For this review, take the finished solid that the model builds, in its own axes (mm). A direction names the side the tool comes from. Coordinates: 2 decimals unless noted, no trailing zeros. Order: outer loops, then holes, each group sorted by start corner. A loop starts at its lowest first (then second) coordinate and runs counter-clockwise, first axis right, second up.
from build123d import *

# Parameters (mm, degrees)
CORTAR_EXTRUIR4_DEPTH      = 312.012057644
SALIENTE_EXTRUIR1_START    = -30
CROQUIS4_R                 = 67.5
SALIENTE_EXTRUIR1_DEPTH    = 30
SALIENTE_EXTRUIR2_START    = 2
CROQUIS5_R                 = 58
CROQUIS5_R_2               = 50.227847336
CROQUIS5_R_3               = 2.860878396
SALIENTE_EXTRUIR2_DEPTH    = 2
CROQUIS6_R                 = 58
SALIENTE_EXTRUIR3_DEPTH    = 73
CORTAR_EXTRUIR5_DEPTH      = 315.148452169
CORTAR_EXTRUIR5_DEPTH_BACK = 315.148452169
CROQUIS7_W                 = 212.825411986
CROQUIS7_H                 = 84.990442804


with BuildPart() as part:
    # Croquis2 → Revolución1 (revolve)
    with BuildSketch(Plane.XY):
        Polygon((0, 0), (-67.5, 0), (-67.5, 26.689315597), (-58, 80), (-58, 296), (0, 296), align=None)
    revolve(axis=Axis((0, 296, 0), (0, -1, 0)))

    # Croquis3 → Cortar-Extruir4 (cut, through all)
    with BuildSketch(Plane(origin=(0, 296, 0), x_dir=(1, 0, 0), z_dir=(0, 1, 0))):
        Polygon((0, 58), (-8.909431544, 66.909431544), (8.909431544, 66.909431544), align=None)
        Polygon((66.909431544, -8.909431544), (58, 0), (66.909431544, 8.909431544), align=None)
        Polygon((-8.909431544, -66.909431544), (0, -58), (8.909431544, -66.909431544), align=None)
        Polygon((-66.909431544, 8.909431544), (-58, 0), (-66.909431544, -8.909431544), align=None)
    extrude(amount=-CORTAR_EXTRUIR4_DEPTH, mode=Mode.SUBTRACT)

    # Croquis4 → Saliente-Extruir1 (add)
    with BuildSketch(Plane.XZ.offset(SALIENTE_EXTRUIR1_START)):
        with Locations(Location((0, 0, 0), (0, 0, 180))):
            Circle(CROQUIS4_R)
    extrude(amount=SALIENTE_EXTRUIR1_DEPTH)

    # Croquis5 → Saliente-Extruir2 (add)
    with BuildSketch(Plane(origin=(0, 296, 0), x_dir=(1, 0, 0), z_dir=(0, 1, 0)).offset(SALIENTE_EXTRUIR2_START)):
        with Locations(Location((0, 0, 0), (0, 0, 180))):
            Circle(CROQUIS5_R)
        with Locations(Location((0, 0, 0), (0, 0, 180))):
            Circle(CROQUIS5_R_2, mode=Mode.SUBTRACT)
        with Locations(Location((0, 54.172847051, 0), (0, 0, 180))):
            Circle(CROQUIS5_R_3, mode=Mode.SUBTRACT)
        with Locations(Location((46.915061741, 27.086423525, 0), (0, 0, 180))):
            Circle(CROQUIS5_R_3, mode=Mode.SUBTRACT)
        with Locations(Location((46.915061741, -27.086423525, 0), (0, 0, 180))):
            Circle(CROQUIS5_R_3, mode=Mode.SUBTRACT)
        with Locations(Location((0, -54.172847051, 0), (0, 0, 180))):
            Circle(CROQUIS5_R_3, mode=Mode.SUBTRACT)
        with Locations(Location((-46.915061741, -27.086423525, 0), (0, 0, 180))):
            Circle(CROQUIS5_R_3, mode=Mode.SUBTRACT)
        with Locations(Location((-46.915061741, 27.086423525, 0), (0, 0, 180))):
            Circle(CROQUIS5_R_3, mode=Mode.SUBTRACT)
    extrude(amount=-SALIENTE_EXTRUIR2_DEPTH)

    # Croquis6 → Saliente-Extruir3 (add)
    with BuildSketch(Plane(origin=(0, 0, 0), x_dir=(0, 0, -1), z_dir=(1, 0, 0))):
        with Locations((0, 230)):
            Circle(CROQUIS6_R)
    extrude(amount=SALIENTE_EXTRUIR3_DEPTH)

    # Croquis7 → Cortar-Extruir5 (cut, two sides: drawn at the far end of the back side and taken through both)
    with BuildSketch(Plane(origin=(0, 0, 0), x_dir=(0, 0, -1), z_dir=(1, 0, 0)).offset(-CORTAR_EXTRUIR5_DEPTH_BACK)):
        with Locations((5.734816491, 37.504778598)):
            Rectangle(CROQUIS7_W, CROQUIS7_H)
    extrude(amount=CORTAR_EXTRUIR5_DEPTH + CORTAR_EXTRUIR5_DEPTH_BACK, mode=Mode.SUBTRACT)


solid = part.part
1. Take a section at C-C, the plane y = 230. Give the boundary of the cut face in (x, z), plus the area to 3 significant figures.
Answer below:
outline: (0, -58) - (73, -58) - (73, 58) - (0, 58) arc R58 ccw to start
area: 13,800 mm2
2. Clearance check with flat-ended pins moving along their axes: pin 1 Ø8 at (x, z) = (-31.5, 1.5) entering from +Y; pin 2 Ø2 at (x, y) = (32, 210) entering from -Z; pin 3 Ø6 at (x, y) = (-26, 125.5) entering from +Z. State where each tip first meets the part, or that it passes through.
Answer below:
pin 1: stops at y = 296
pin 2: stops at z = -54.8
pin 3: stops at z = 53.24
3. Take a section at D-D, the plane x = -35. Give the boundary of the cut face in (y, z).
Answer below:
outline: (80, -46.25) - (298, -46.25) - (298, -36.03) - (296, -36.03) - (296, 36.03) - (298, 36.03) - (298, 46.25) - (80, 46.25) - close
4. Take a section at A-A, the plane z = 0. Give the boundary of the cut face in (x, y).
Answer below:
outline: (-58, 80) - (58, 80) - (58, 172) - (73, 172) - (73, 288) - (58, 288) - (58, 298) - (50.23, 298) - (50.23, 296) - (-50.23, 296) - (-50.23, 298) - (-58, 298) - close
5. Machinability: for faces 4 (the face through (0, 296, 54)), 5 (the face through (52.211, 232.55, 57.944)), 6 (the face through (73, 231, 1)), which of the approach directions +Z, -Z, +X, -X, +Y, -Y give a long, thin tool a straight path to every point of the face, cutting with its end or side? Answer none if there is none.
Answer below:
face 4: +Y
face 5: +X
face 6: +Z, -Z, +X, +Y, -Y
6. The part is to be moulded in two halves that separate along X. For faces 1 (the face through (48, 298, -17)), 2 (the face through (50.18, 297.01, 2.21)), 3 (the face through (-55.322, 190.526, -17.422)), say which applies: +X half, -X half, draft (parallel to the pull), parting line (faces both ways), or undercut.
Answer below:
face 1: draft
face 2: undercut
face 3: parting line
7. To check wall thickness, follow L1, parallel to Z at x = 0, y = 297.4; L2, parallel to Y at x = 17.5, z = -11.5; L3, parallel to Z at x = -16, y = 211. State the ranges of each line that lie inside material, in increasing order.
Answer below:
L1: z = -58 to -57.03, -51.31 to -50.23, 50.23 to 51.31, 57.03 to 58
L2: y = 80 to 296
L3: z = -55.75 to 55.75
8. Take a section at B-B, the plane x = 40. Give the boundary of the cut face in (y, z).
Answer below:
outline: (80, -42) - (190, -42) arc R58 ccw to (270, -42) - (298, -42) - (298, -30.38) - (296, -30.38) - (296, 30.38) - (298, 30.38) - (298, 42) - (270, 42) arc R58 ccw to (190, 42) - (80, 42) - close
